Part model, mm, in its own coordinate system. A direction names the side the tool comes from. Round coordinates to 2 decimals unless told otherwise and drop trailing zeros. Write each loop counter-clockwise with the first axis right and the second up, starting at its lowest first coordinate (ties: lowest second). Pieces come first, ordered by that corner, then holes. Notation, with made-up numbers: M 30.25,3 L 53.25,3 A13 cw 53.25,28 Z; hole C -37.5,-27.5 d5. An arc over 180 degrees is marked long. Answer as a JSON object with one key per item and string values. Group by question number.
1. Drill centre lines: line 1 (Y direction, x = 0, z = 6) (3 decimals); line 2 (Z direction, x = 1.45, y = 0). Where is each one in solid material? Low to high. Write a range as from..to.
2. Which spindle directions (+Z, -Z, +X, -X, +Y, -Y) get a long thin tool onto all of the face, cutting with end or side? Do faces 1 (the face through (0, 0, 12)), 2 (the face through (1, -1, 10.4)). Say none if no direction does.
3. Drop flat-ended pins along their axis: pin 1 (1.5 mm diameter, centred on x = 1, y = 0, fed in from -Z); pin 2 (1 mm diameter, centred on x = -1, z = 8, fed in from -Y); pin 3 (1 mm diameter, centred on y = -0.5, z = 6, fed in from +X) (3 decimals). Give the stop position or say it passes through.
4. Band-saw the part on A-A, the plane z = 3.5. Write the cut outline in (x, y) (3 decimals).
from build123d import *

# Parameters (mm, degrees)
ESBO_O1_R                = 1.125
RESSALTO_EXTRUS_O1_DEPTH = 12
ESBO_O2_R                = 2.125
RESSALTO_EXTRUS_O2_DEPTH = 1.6
FILETE1_R                = 1.6


with BuildPart() as part:
    # Esboço1 → Ressalto-extrusão1 (new body)
    with BuildSketch(Plane.XY):
        Circle(ESBO_O1_R)
    extrude(amount=RESSALTO_EXTRUS_O1_DEPTH)

    # Esboço2 → Ressalto-extrusão2 (add)
    with BuildSketch(Plane.XY.offset(12)):
        Circle(ESBO_O2_R)
    extrude(amount=-RESSALTO_EXTRUS_O2_DEPTH)

    # Filete1
    filete1_edges = [part.edges().sort_by_distance(p)[0] for p in [
        (-2.125, 0, 12),
    ]]
    fillet(filete1_edges, radius=FILETE1_R - 0.0001)  # a hair under: the kernel refuses the full size


solid = part.part
Worked answers:
{
 "1": {"line 1": "y = -1.125..1.125", "line 2": "z = 10.4..11.71"},
 "2": {"face 1": "+Z, +X, -X, +Y, -Y", "face 2": "-Z"},
 "3": {"pin 1": "stops at z = 0", "pin 2": "stops at y = -1.01", "pin 3": "stops at x = 1.125"},
 "4": {"outline": "C 0,0 d2.25"}
}
